CAD build for the part. Positions are in the model's coordinates, mm. A direction names the side the tool comes from. Coordinates: 2 decimals unless noted, no trailing zeros. Write each loop counter-clockwise with the first axis right and the second up, starting at its lowest first coordinate (ties: lowest second). Pieces come first, ordered by that corner, then holes. Notation, with made-up numbers: (11, -27) -> (37, -27) arc R27 cw to (37, -8) -> close; hole circle Ø2 at (36, -23). An arc over 180 degrees is marked (long way). Answer as CSV lines item,"result". Start each with the question number.
```python
from build123d import *

# Parameters (mm, degrees)
SKETCH_1_R               = 1.9
EXTRUDE_1_DEPTH          = 20
SKETCH_2_W               = 37.909545504
SKETCH_2_H               = 0.4
EXTRUDE_2_DEPTH          = 20
EXTRUDE_2_DEPTH_BACK     = 40
FILLET_1_R               = 15
FILLET_2_R               = 5
FILLET_3_R               = 3
CUT_EXTRUDE_1_DEPTH      = 20
SKETCH_4_W               = 8
SKETCH_4_H               = 4.180908992
CUT_EXTRUDE_2_DEPTH      = 2.9
CUT_EXTRUDE_2_DEPTH_BACK = 3.3


with BuildPart() as part:
    # 草图1 → 凸台-拉伸1 (new body)
    with BuildSketch(Plane(origin=(0, 0, 0), x_dir=(0, 0, -1), z_dir=(1, 0, 0))):
        with BuildLine():
            Line((-10, -0.2), (-2.090454496, -0.2))
            ThreePointArc((-2.090454496, -0.2), (0, -2.1), (2.090454496, -0.2))
            Line((2.090454496, -0.2), (40, -0.2))
            Line((40, -0.2), (40, 0.2))
            Line((40, 0.2), (2.090454496, 0.2))
            ThreePointArc((2.090454496, 0.2), (0, 2.1), (-2.090454496, 0.2))
            Line((-2.090454496, 0.2), (-10, 0.2))
            Line((-10, 0.2), (-10, -0.2))
        make_face()
        Circle(SKETCH_1_R, mode=Mode.SUBTRACT)
    extrude(amount=EXTRUDE_1_DEPTH)

    # 草图2 → 凸台-拉伸2 (add, two sides)
    with BuildSketch(Plane(origin=(20, 0, 0), x_dir=(0, 0, -1), z_dir=(1, 0, 0))) as extrude_2_sk:
        with Locations((21.045227248, 0)):
            Rectangle(SKETCH_2_W, SKETCH_2_H)
    extrude(amount=EXTRUDE_2_DEPTH)
    extrude(extrude_2_sk.sketch, amount=-EXTRUDE_2_DEPTH_BACK)

    # 圆角1
    fillet_1_edges = [part.edges().sort_by_distance(p)[0] for p in [
        (-20, 0, -40),
        (40, 0, -40),
    ]]
    fillet(fillet_1_edges, radius=FILLET_1_R)

    # 圆角2
    fillet_2_edges = [part.edges().sort_by_distance(p)[0] for p in [
        (-20, 0, -2.090454496),
        (40, 0, -2.090454496),
    ]]
    fillet(fillet_2_edges, radius=FILLET_2_R)

    # 圆角3
    fillet_3_edges = [part.edges().sort_by_distance(p)[0] for p in [
        (0, 0, 10),
        (20, 0, 10),
    ]]
    fillet(fillet_3_edges, radius=FILLET_3_R)

    # 草图3 → 切除-拉伸1 (cut)
    with BuildSketch(Plane(origin=(0, 0.2, 0), x_dir=(1, 0, 0), z_dir=(0, 1, 0))):
        with BuildLine():
            ThreePointArc((11.25, -7), (10.883883476, -6.116116524), (10, -5.75))
            Line((10, -5.75), (10, -8.25))
            ThreePointArc((10, -8.25), (10.883883476, -7.883883476), (11.25, -7))
        make_face()
        with BuildLine():
            Line((10, -8.25), (10, -5.75))
            ThreePointArc((10, -5.75), (8.75, -7), (10, -8.25))
        make_face()
    extrude(amount=-CUT_EXTRUDE_1_DEPTH, mode=Mode.SUBTRACT)

    # 草图4 → 切除-拉伸2 (cut, two sides)
    with BuildSketch(Plane(origin=(0, 0.2, 0), x_dir=(1, 0, 0), z_dir=(0, 1, 0))) as cut_extrude_2_sk:
        with Locations((10, 0)):
            Rectangle(SKETCH_4_W, SKETCH_4_H)
    extrude(amount=CUT_EXTRUDE_2_DEPTH, mode=Mode.SUBTRACT)
    extrude(cut_extrude_2_sk.sketch, amount=-CUT_EXTRUDE_2_DEPTH_BACK, mode=Mode.SUBTRACT)


solid = part.part
```
1. Tool access for faces 1 (the face through (0, 0, 2.1)), 2 (the face through (10, 0.2, 5)), 3 (the face through (10, -0.2, -21)): list every direction of +Z, -Z, +X, -X, +Y, -Y with a clear straight run to the whole face (end or side of a thin tool).
2. Cut at A-A (z = 0). Give the cut face in (x, y), then the cut area to 3 significant figures.
3. Cut at D-D (x = -16). Give the cut face in (y, z), then the cut area to 3 significant figures.
4. Wall check: line 1 (Y direction, x = 15, z = 0); line 2 (Y direction, x = 23, z = -5.5); line 3 (Z direction, x = 15.85, y = 0). Give the ranges that are in metal, low to high.
5. Flat gauge pins, fed straight in: P1, Ø2, axis at y = 0, z = -1, coming from the -X side; P2, Ø2, axis at y = 0.5, z = 0, coming from the +X side; P3, Ø12, axis at x = -11, z = -28, coming from the -Y side; P4, Ø3, axis at x = 20, z = -19, coming from the +Y side. Where does each tip first touch, or does it go through?
6. Cut at B-B (y = -1.1). Give the cut face in (x, z).
7. Cut at C-C (z = -16.5). Give the cut face in (x, y).
Geometry check:
1,face 1,"+Z, -X, +Y, -Y"
1,face 2,"+Z, +X, -X, +Y"
1,face 3,"-Z, +X, -X, -Y"
2,outline,"(0, -2.1) -> (6, -2.1) -> (6, -1.9) -> (0, -1.9) -> close; (0, 1.9) -> (6, 1.9) -> (6, 2.1) -> (0, 2.1) -> close; (14, -2.1) -> (20, -2.1) -> (20, -1.9) -> (14, -1.9) -> close; (14, 1.9) -> (20, 1.9) -> (20, 2.1) -> (14, 2.1) -> close"
2,area,"4.80 mm²"
3,outline,"(-0.2, -35.2) -> (0.2, -35.2) -> (0.2, -2.19) -> (-0.2, -2.19) -> close"
3,area,"13.2 mm²"
4,line 1,"-2.1 to -1.9, 1.9 to 2.1"
4,line 2,"-0.2 to 0.2"
4,line 3,"-40 to -1.9, 1.9 to 10"
5,P1,"x = 0"
5,P2,"through"
5,P3,"y = -0.2"
5,P4,"y = 0.2"
6,outline,"(0, -1.79) -> (6, -1.79) -> (6, -1.55) -> (0, -1.55) -> close; (0, 1.55) -> (6, 1.55) -> (6, 1.79) -> (0, 1.79) -> close; (14, -1.79) -> (20, -1.79) -> (20, -1.55) -> (14, -1.55) -> close; (14, 1.55) -> (20, 1.55) -> (20, 1.79) -> (14, 1.79) -> close"
7,outline,"(-20, -0.2) -> (40, -0.2) -> (40, 0.2) -> (-20, 0.2) -> close"
